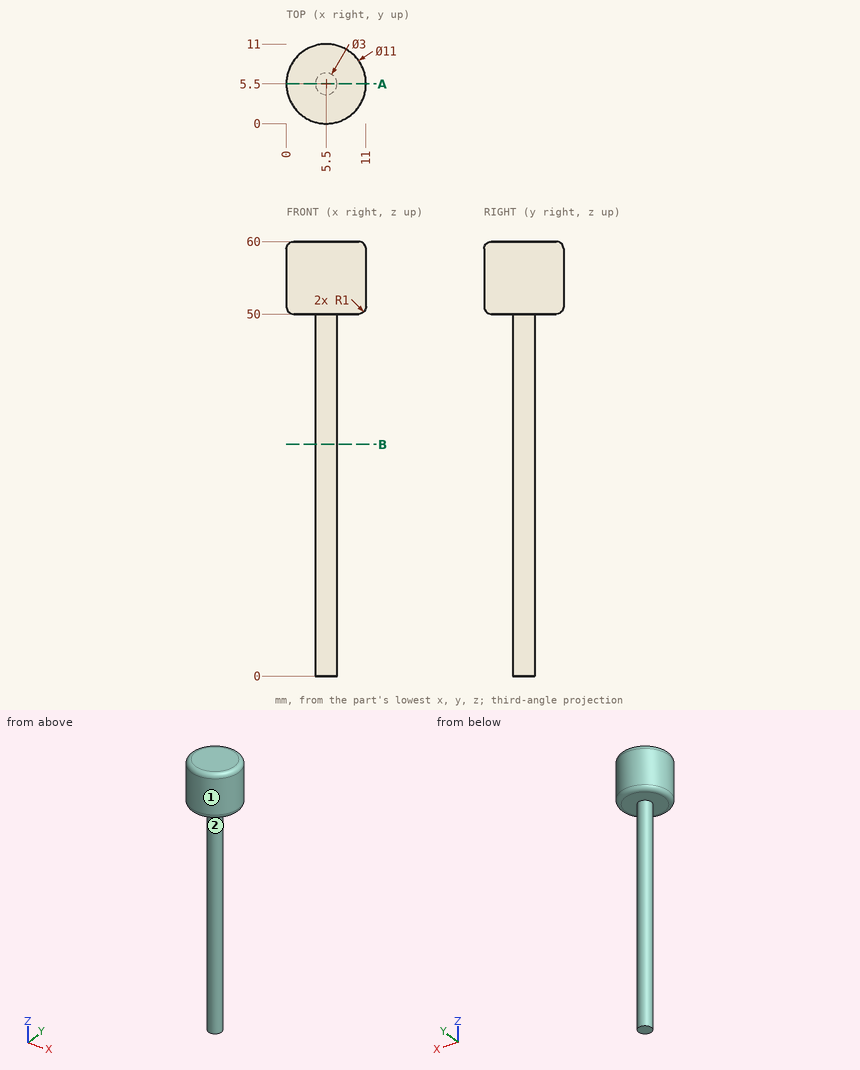
Geometry check sheet. Reference: drawing and pictorial views, mm from the part's lowest x, y, z. A direction names the side the tool comes from. Give positions to 0.01 mm unless a question says otherwise; leave off trailing zeros. Order: outer loops, then holes, each group sorted by start corner. A loop starts at its lowest first (then second) coordinate and runs counter-clockwise, first axis right, second up. Notation, with made-up numbers: M 41.25,60 L 82.25,60 A20 ccw 82.25,94 Z; hole C -12,12.25 d2. An arc over 180 degrees is marked long. Use one line per item in the form item = value. Start each with the question number.
Q1. Section check B-B (z = 32). Enter the section's corners in (x, y), then the cut area to 3 significant figures.
Q2. Section check A-A (y = 5.5). Enter the section's corners in (x, z), then the cut area to 3 significant figures.
Q3. Access from +Z, -Z, +X, -X, +Y, -Y to the whole of each face (thin tool, end or side, straight path). Record for the marked faces 1 and 2.
Q4. Go/stop test with flat-tipped pins: pin 1 Ø5 at (x, z) = (8.5, 8) entering from -Y; pin 2 Ø6 at (y, z) = (6.5, 22) entering from -X; pin 3 Ø2 at (x, z) = (7.5, 39) entering from +Y. Record where each tip stops, or that it passes through.
Q5. Scan lines: line 1 along Z through (x, y) = (1.5, 6.75); line 2 along Y through (x, z) = (5.5, 23); line 3 along X through (y, z) = (2, 51.5). Record each from-to range of solid material in increasing order. Write a range as [from, to].
Evaluation:
q1.outline = C 5.5,5.5 d3
q1.area = 7.07 mm2
q2.outline = M 0,51 A1 ccw 1,50 L 4,50 L 4,0 L 7,0 L 7,50 L 10,50 A1 ccw 11,51 L 11,59 A1 ccw 10,60 L 1,60 A1 ccw 0,59 Z
q2.area = 259 mm2
q3.face_1 = +Z, -Z
q3.face_2 = -Z
q4.pin_1 = 4.09
q4.pin_2 = 4
q4.pin_3 = 6.62
q5.line_1 = [50, 60]
q5.line_2 = [4, 7]
q5.line_3 = [1.26, 9.74]
